Work out the finished part from the listing and answer in its coordinate system (mm). Face numbers are marked on the shaded views. A direction names the side the tool comes from. Round coordinates to 2 decimals unless told otherwise and drop trailing zeros. Write each loop counter-clockwise with the first axis right and the second up, starting at its lowest first coordinate (ties: lowest second). Pieces come first, ordered by that corner, then holes. Notation, with made-up numbers: (22, -0.75) - (30, -0.75) arc R27 ccw to (30, 23.25) - close; hole circle Ø4 at (37.25, 74.5). An arc over 180 degrees is marked (long way). Write item = value, one per line. Start each with the question number.
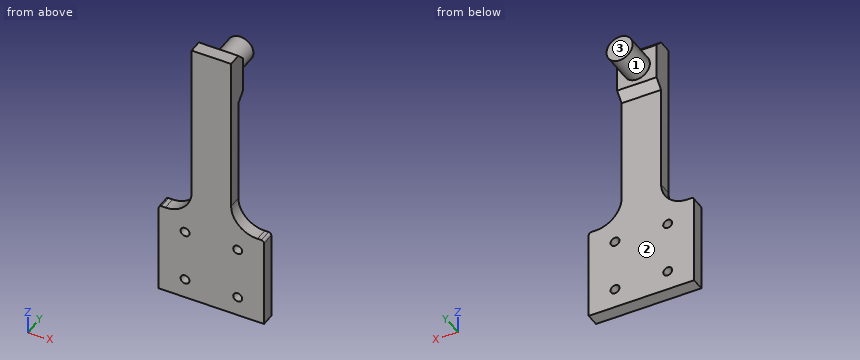
from build123d import *

# Parameters (mm, degrees)
SKETCH1_W                    = 40
SKETCH1_H                    = 35
BOSS_EXTRUDE1_DEPTH          = 5
M3_CLEARANCE_HOLE1_OUTLINE_R = 1.7
M3_CLEARANCE_HOLE1_DEPTH     = 5
SKETCH7_W                    = 15
SKETCH7_H                    = 70
BOSS_EXTRUDE3_DEPTH          = 5
SKETCH8_R                    = 4.96
BOSS_EXTRUDE4_DEPTH          = 15
SKETCH9_W                    = 15
SKETCH9_H                    = 12
BOSS_EXTRUDE5_DEPTH          = 3.15
FILLET1_R                    = 10
FILLET2_R                    = 1
CHAMFER1_SIZE                = 4


# Read off the part's stored shape, not the designer's step: M3 Clearance Hole1
with BuildPart() as part:
    # Sketch1 → Boss-Extrude1 (new body)
    with BuildSketch(Plane(origin=(0, 0, 0), x_dir=(1, 0, 0), z_dir=(0, 1, 0))):
        Rectangle(SKETCH1_W, SKETCH1_H)
    extrude(amount=BOSS_EXTRUDE1_DEPTH)

    # M3 Clearance Hole1 outline → M3 Clearance Hole1 (cut)
    with BuildSketch(Plane(origin=(0, 0, 0), x_dir=(1, 0, 0), z_dir=(0, 1, 0))):
        with Locations((10, 10)):
            Circle(M3_CLEARANCE_HOLE1_OUTLINE_R)
        with Locations((-10, -10)):
            Circle(M3_CLEARANCE_HOLE1_OUTLINE_R)
        with Locations((-10, 10)):
            Circle(M3_CLEARANCE_HOLE1_OUTLINE_R)
        with Locations((10, -10)):
            Circle(M3_CLEARANCE_HOLE1_OUTLINE_R)
    extrude(amount=M3_CLEARANCE_HOLE1_DEPTH, mode=Mode.SUBTRACT)

    # Sketch7 → Boss-Extrude3 (add, through all)
    with BuildSketch(Plane(origin=(0, 5, 0), x_dir=(1, 0, 0), z_dir=(0, 1, 0))):
        with Locations((0, -52.5)):
            Rectangle(SKETCH7_W, SKETCH7_H)
    extrude(amount=-BOSS_EXTRUDE3_DEPTH)

    # Sketch8 → Boss-Extrude4 (add)
    with BuildSketch(Plane(origin=(0, 5, 0), x_dir=(1, 0, 0), z_dir=(0, 1, 0))):
        with Locations(Location((0, -77.5, 0), (0, 0, 270))):
            Circle(SKETCH8_R)
    extrude(amount=BOSS_EXTRUDE4_DEPTH)

    # Sketch9 → Boss-Extrude5 (add)
    with BuildSketch(Plane(origin=(0, 5, 0), x_dir=(1, 0, 0), z_dir=(0, 1, 0))):
        with Locations((0, -77.5)):
            Rectangle(SKETCH9_W, SKETCH9_H)
    extrude(amount=BOSS_EXTRUDE5_DEPTH)

    # Fillet1
    fillet1_edges = [part.edges().sort_by_distance(p)[0] for p in [
        (-7.5, 2.5, 17.5),
        (7.5, 2.5, 17.5),
    ]]
    fillet(fillet1_edges, radius=FILLET1_R)

    # Fillet2
    fillet2_edges = [part.edges().sort_by_distance(p)[0] for p in [
        (20, 2.5, 17.5),
        (-20, 2.5, 17.5),
    ]]
    fillet(fillet2_edges, radius=FILLET2_R)

    # Chamfer1
    # the kernel refuses this chamfer: 4 mm, written as the material it adds along each edge
    with BuildSketch(Plane(origin=(7.5, 5, 71.5), x_dir=(0, -0.027495876610586296, -0.9996219169112968), z_dir=(-1, 0, 0))) as chamfer1_piece_1_section:
        Polygon((CHAMFER1_SIZE * 0.999621916911, -CHAMFER1_SIZE * 0.0274958766106), (-CHAMFER1_SIZE * 0.0274958766106, -CHAMFER1_SIZE * 0.999621916911), (0, 0), align=None)
    chamfer1_piece_1 = extrude(amount=15, mode=Mode.PRIVATE)
    chamfer1_piece_1 = split(chamfer1_piece_1, bisect_by=Plane(origin=(0, 8.15, 70.111191503), z_dir=(0, -1, 0)), keep=Keep.TOP, mode=Mode.PRIVATE)
    add(chamfer1_piece_1)
    with BuildSketch(Plane(origin=(-7.5, 5, 83.5), x_dir=(0, -0.027495876610586296, 0.9996219169112968), z_dir=(1, 0, 0))) as chamfer1_piece_2_section:
        Polygon((CHAMFER1_SIZE * 0.999621916911, -CHAMFER1_SIZE * 0.0274958766106), (-CHAMFER1_SIZE * 0.0274958766106, -CHAMFER1_SIZE * 0.999621916911), (0, 0), align=None)
    chamfer1_piece_2 = extrude(amount=15, mode=Mode.PRIVATE)
    chamfer1_piece_2 = split(chamfer1_piece_2, bisect_by=Plane(origin=(0, 6.188699504, 87.5), z_dir=(0, 0, -1)), keep=Keep.TOP, mode=Mode.PRIVATE)
    chamfer1_piece_2 = split(chamfer1_piece_2, bisect_by=Plane(origin=(0, 8.15, 84.884013224), z_dir=(0, -1, 0)), keep=Keep.TOP, mode=Mode.PRIVATE)
    add(chamfer1_piece_2)


solid = part.part
1. Consider line 1 (Z direction, x = 10, y = 3.05); line 2 (X direction, y = 1.75, z = 10); line 3 (Z direction, x = 0, y = 11). Determine where each line is inside the solid, lowest interval first.
2. Find section A-A on z = -10. Give the vertices of the cut face in (x, y).
3. Each of these flat-tipped pins is pushed along its axis until it touches: pin 1 (8 mm diameter, centred on x = -6.5, z = 52.5, fed in from -Y); pin 2 (1.2 mm diameter, centred on x = -18, y = 3, fed in from +Z); pin 3 (8 mm diameter, centred on x = -12.5, y = 9.5, fed in from +Z); pin 4 (2.5 mm diameter, centred on y = 3.5, z = 60.5, fed in from +X). Where does it stop, or does it pass through?
4. Which of the six approach directions +Z, -Z, +X, -X, +Y, -Y give full straight-line access (tool end or side, diameter ignored) to the marked faces 1, 2 and 3?
5. Find section C-C on x = 10. Give the vertices of the cut face in (y, z), plus the area to 3 significant figures.
6. Find section B-B on x = 0. Give the vertices of the cut face in (y, z).
7. Find section D-D on z = 77.5. Give the vertices of the cut face in (x, y), plus the area to 3 significant figures.
Answer key:
q1.line_1 = -17.5 to -11.7, -8.3 to 8.3, 11.7 to 20.89
q1.line_2 = -20 to -11.7, -8.3 to 8.3, 11.7 to 20
q1.line_3 = 72.54 to 82.46
q2.outline = (-20, 0) - (-11.7, 0) - (-11.7, 5) - (-20, 5) - close; (-8.3, 0) - (8.3, 0) - (8.3, 5) - (-8.3, 5) - close; (11.7, 0) - (20, 0) - (20, 5) - (11.7, 5) - close
q3.pin_1 = 0
q3.pin_2 = 17.5
q3.pin_3 = through
q3.pin_4 = 7.5
q4.face_1 = +Y
q4.face_2 = -Z, +X, -X, +Y
q4.face_3 = +Z, -Z, +X, -X, +Y
q5.outline = (0, -17.5) - (5, -17.5) - (5, -11.7) - (0, -11.7) - close; (0, -8.3) - (5, -8.3) - (5, 8.3) - (0, 8.3) - close; (0, 11.7) - (5, 11.7) - (5, 20.89) - (0, 20.89) - close
q5.area = 158 mm²
q6.outline = (0, -17.5) - (5, -17.5) - (5, 67.5) - (8.15, 70.65) - (8.15, 72.54) - (20, 72.54) - (20, 82.46) - (8.15, 82.46) - (8.15, 84.35) - (5, 87.5) - (0, 87.5) - close
q7.outline = (-7.5, 0) - (7.5, 0) - (7.5, 8.15) - (4.96, 8.15) - (4.96, 20) - (-4.96, 20) - (-4.96, 8.15) - (-7.5, 8.15) - close
q7.area = 240 mm²
